```python
from build123d import *

# Parameters (mm, degrees)
MAIN_BLOCK_SKETCH_W          = 70
MAIN_BLOCK_SKETCH_H          = 20
MAIN_BLOCK_DEPTH             = 25
THICKER_SECTION_SKETCH_W     = 32
THICKER_SECTION_SKETCH_H     = 20
THICKER_SECTION_DEPTH        = 5
BELT_TRAP_CUT_SKETCH_W       = 6
BELT_TRAP_CUT_SKETCH_H       = 2.5
BELT_TRAP_CUT_DEPTH          = 45.158804332
BELT_HOLDER_MOUNTING_HOLES_D = 3.4
NUT_TRAPS_DEPTH              = 2.3
MOUNTING_HOLES_D             = 5.5
MOUNTING_HOLES_CBORE_D       = 10
MOUNTING_HOLES_CBORE_DEPTH   = 5.4
PRINT_HELPER_FILLETS_R       = 1
BELT_GUIDE_CHAMFERS_SIZE     = 1
COSMETIC_CHAMFERS_SIZE       = 1


with BuildPart() as part:
    # Main Block Sketch → Main Block (new body)
    with BuildSketch(Plane.XY):
        Rectangle(MAIN_BLOCK_SKETCH_W, MAIN_BLOCK_SKETCH_H)
    extrude(amount=MAIN_BLOCK_DEPTH)

    # Thicker Section Sketch → Thicker Section (add)
    with BuildSketch(Plane.XY.offset(25)):
        with Locations((19, 0)):
            Rectangle(THICKER_SECTION_SKETCH_W, THICKER_SECTION_SKETCH_H)
        with Locations((-19, 0)):
            Rectangle(THICKER_SECTION_SKETCH_W, THICKER_SECTION_SKETCH_H)
    extrude(amount=THICKER_SECTION_DEPTH)

    # Belt Trap Cut Sketch → Belt Trap Cut (cut, through all)
    with BuildSketch(Plane.XY.offset(25)):
        Rectangle(BELT_TRAP_CUT_SKETCH_W, BELT_TRAP_CUT_SKETCH_H)
    extrude(amount=-BELT_TRAP_CUT_DEPTH, mode=Mode.SUBTRACT)

    # Belt Holder Mounting Holes (through all)
    with Locations(Plane.XY.offset(30)):
        with Locations((-10, 5), (10, 5), (-10, -5), (10, -5)):
            Hole(BELT_HOLDER_MOUNTING_HOLES_D / 2)

    # Nut Trap Sketch → Nut Traps (cut)
    with BuildSketch(Plane.XY):
        Polygon((11.558845727, 7.7), (8.441154273, 7.7), (6.882308546, 5), (8.441154273, 2.3), (11.558845727, 2.3), (13.117691454, 5), align=None)
        Polygon((-11.558845727, 7.7), (-13.117691454, 5), (-11.558845727, 2.3), (-8.441154273, 2.3), (-6.882308546, 5), (-8.441154273, 7.7), align=None)
        Polygon((-8.441154273, -7.7), (-11.558845727, -7.7), (-13.117691454, -5), (-11.558845727, -2.3), (-8.441154273, -2.3), (-6.882308546, -5), align=None)
        Polygon((13.117691454, -5), (11.558845727, -7.7), (8.441154273, -7.7), (6.882308546, -5), (8.441154273, -2.3), (11.558845727, -2.3), align=None)
    extrude(amount=NUT_TRAPS_DEPTH, mode=Mode.SUBTRACT)

    # Mounting Holes (through all)
    with Locations(Plane(origin=(0, -10, 0), x_dir=(-1, 0, 0), z_dir=(0, -1, 0))):
        with Locations((-25, -10), (25, -10)):
            CounterBoreHole(MOUNTING_HOLES_D / 2, MOUNTING_HOLES_CBORE_D / 2, MOUNTING_HOLES_CBORE_DEPTH)

    # Print Helper Fillets
    print_helper_fillets_edges = [part.edges().sort_by_distance(p)[0] for p in [
        (-3, -10, 27.5),
        (-35, 10, 15),
        (-3, 10, 27.5),
        (-35, -10, 15),
        (3, 10, 27.5),
        (3, -10, 27.5),
        (35, -10, 15),
        (35, 10, 15),
    ]]
    fillet(print_helper_fillets_edges, radius=PRINT_HELPER_FILLETS_R)

    # Belt Guide Chamfers
    belt_guide_chamfers_edges = [part.edges().sort_by_distance(p)[0] for p in [
        (0, 1.25, 25),
        (0, -1.25, 25),
    ]]
    chamfer(belt_guide_chamfers_edges, length=BELT_GUIDE_CHAMFERS_SIZE)

    # Cosmetic Chamfers
    cosmetic_chamfers_edges = [part.edges().sort_by_distance(p)[0] for p in [
        (-3, 0, 30),
        (-19, -10, 30),
        (19, -10, 30),
        (-19, 10, 30),
        (-35, 0, 30),
        (-34.707106781, 9.707106781, 30),
        (-34.707106781, -9.707106781, 30),
        (-3.292893219, 9.707106781, 30),
        (-3.292893219, -9.707106781, 30),
        (3, 0, 30),
        (35, 0, 30),
        (19, 10, 30),
        (34.707106781, 9.707106781, 30),
        (34.707106781, -9.707106781, 30),
        (3.292893219, 9.707106781, 30),
        (3.292893219, -9.707106781, 30),
    ]]
    chamfer(cosmetic_chamfers_edges, length=COSMETIC_CHAMFERS_SIZE)


solid = part.part
```
Source: CAD feature listing. Evaluate the final solid. Frame: model axes, mm. A direction names the side the tool comes from. Coordinates: 2 decimals unless noted, no trailing zeros. Loops run counter-clockwise (first coordinate to the right, second up) from the corner with the lowest first, then second, coordinate; pieces in that order, holes last. Notation, with made-up numbers: M 58,16 L 99,16 A26 cw 99,46 Z; hole C 60,66 d3. An arc over 180 degrees is marked long. Put each result on its own line as item: value. Start each with the question number.
1) Pull-direction query (Z, two-part tool) for faces 4 (the face through (-20, -7, 10)), 5 (the face through (7.65, 3.67, 1.13)), 6 (the face through (-19, 0, 30)); classes: pulls with the +Z half, pulls with the -Z half, needs draft (parallel to the pull), parting line crosses it, or undercut.
2) Ray query, L1, parallel to X at y = 2.25, z = 10; L2, parallel to Y at x = 10, z = 16.25; L3, parallel to Z at x = 25, y = -7.9. Return the intervals inside material, ascending. Write a range as from..to.
3) Contact query for flat-ended pins moving along their axis: pin 1 Ø8 at (x, z) = (25, 10) entering from +Y; pin 2 Ø9 at (x, z) = (-25, 10) entering from -Y. Output: stop coordinate, or through.
4) Reachability of faces 1 (the face through (-10, 7.7, 1)), 2 (the face through (9.2, 3.5, 16)), 3 (the face through (-3, -1, 21)) from +Z, -Z, +X, -X, +Y, -Y: full face, straight path, thin tool, end or side. Return the list, or none.
5) Cut plane B-B on y = 4. Give the number of separate pieces and of enclosed holes in the cut face, then the cut area to 3 significant figures.
6) Cut plane C-C on z = 18.5. Return the cut outline in (x, y), then the cut area to 3 significant figures.
7) Cut plane A-A on x = -10. Return the cut outline in (y, z).
The answers:
1. face 4: undercut
1. face 5: needs draft
1. face 6: pulls with the +Z half
2. L1: x = -35..-27.75, -22.25..22.25, 27.75..35
2. L2: y = -10..-6.7, -3.3..3.3, 6.7..10
2. L3: z = 0..5, 15..30
3. pin 1: stops at y = 10
3. pin 2: stops at y = -4.6
4. face 1: -Z
4. face 2: +Z, -Z
4. face 3: +Z
5. separate pieces: 3
5. enclosed holes: 2
5. area: 1,840 mm²
6. outline: M -35,-9 A1 ccw -34,-10 L 34,-10 A1 ccw 35,-9 L 35,9 A1 ccw 34,10 L -34,10 A1 ccw -35,9 Z; hole C -10,-5 d3.4; hole C -10,5 d3.4; hole M -3,-1.25 L 3,-1.25 L 3,1.25 L -3,1.25 Z; hole C 10,-5 d3.4; hole C 10,5 d3.4
6. area: 1,350 mm²
7. outline: M -10,0 L -7.7,0 L -7.7,2.3 L -6.7,2.3 L -6.7,30 L -9,30 L -10,29 Z; M -3.3,2.3 L -2.3,2.3 L -2.3,0 L 2.3,0 L 2.3,2.3 L 3.3,2.3 L 3.3,30 L -3.3,30 Z; M 6.7,2.3 L 7.7,2.3 L 7.7,0 L 10,0 L 10,29 L 9,30 L 6.7,30 Z
